Study the drawing (mm; zero at the part's minimum x, y, z) and answer. A direction names the side the tool comes from. Coordinates: 2 decimals unless noted, no trailing zeros. Loops run counter-clockwise (first coordinate to the right, second up) from the corner with the lowest first, then second, coordinate; pieces in that order, holes last. Notation, with made-up numbers: (63.25, 78.5) - (95.25, 78.5) arc R28 ccw to (95.25, 108.5) - close; hole circle Ø11 at (-1, 10). An arc over 180 degrees is marked (long way). Use one line per item in the form item = value.
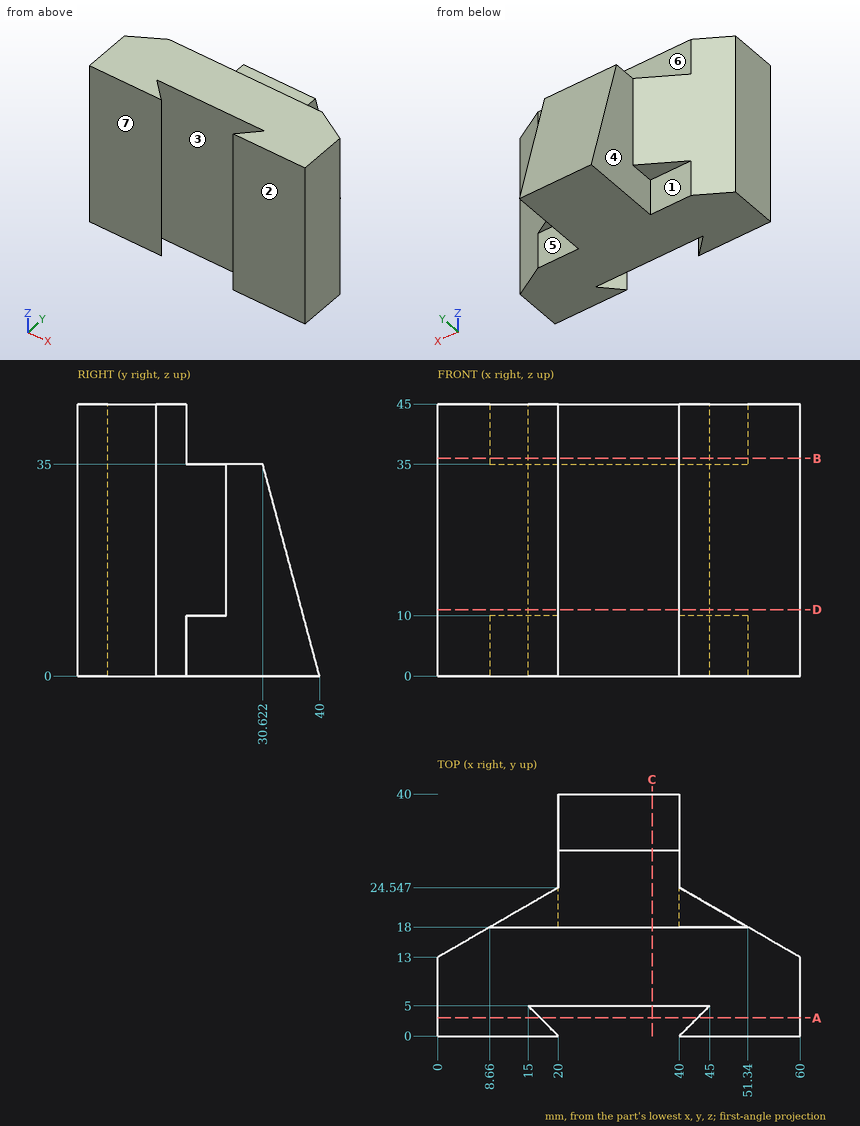
Item 1: The part is cut by section D-D on z = 11. Give the vertices of the cut face in (x, y).
Results below:
outline = (0, 0) - (20, 0) - (15, 5) - (45, 5) - (40, 0) - (60, 0) - (60, 13) - (40, 24.55) - (40, 37.05) - (20, 37.05) - (20, 24.55) - (0, 13) - close
Item 2: Each of these flat-tipped pins is pushed along its axis until it touches: P1, Ø2, axis at x = 46, y = 21.5, coming from the +Z side; P2, Ø1.5, axis at x = 11, z = 20, coming from the +Y side; P3, Ø17.5, axis at y = 28.5, z = 19.5, coming from the +X side. Where does it stop, or does it pass through?
Results below:
P1 = 35
P2 = 19.78
P3 = 48.31
Item 3: Which of the six approach directions +Z, -Z, +X, -X, +Y, -Y give full straight-line access (tool end or side, diameter ignored) to the marked faces 5, 6 and 7?
Results below:
face_5 = -Z, +X, +Y
face_6 = +Z, +X, -X, +Y
face_7 = +Z, -Z, +X, -X, -Y
Item 4: The part is cut by section C-C on x = 35.5. Give the vertices of the cut face in (y, z).
Results below:
outline = (5, 0) - (40, 0) - (30.62, 35) - (18, 35) - (18, 45) - (5, 45) - close
Item 5: The part is cut by section B-B on z = 36. Give the vertices of the cut face in (x, y).
Results below:
outline = (0, 0) - (20, 0) - (15, 5) - (45, 5) - (40, 0) - (60, 0) - (60, 13) - (51.34, 18) - (8.66, 18) - (0, 13) - close
Item 6: For a pull along Y with two mould halves and no side action, classify the marked faces 1, 2, 3 and 4 as +Y half, -Y half, draft (parallel to the pull), parting line (faces both ways), or undercut.
Results below:
face_1 = +Y half
face_2 = -Y half
face_3 = undercut
face_4 = draft
Item 7: Find the intervals of material crossed by L1, parallel to Y at x = 38.5, z = 40; L2, parallel to X at y = 2.5, z = 23; L3, parallel to Y at x = 44, z = 3, in increasing order.
Results below:
L1 = 5 to 18
L2 = 0 to 17.5, 42.5 to 60
L3 = 0 to 4, 5 to 18
Item 8: The part is cut by section A-A on y = 3. Give the vertices of the cut face in (x, z).
Results below:
outline = (0, 0) - (17, 0) - (17, 45) - (0, 45) - close; (43, 0) - (60, 0) - (60, 45) - (43, 45) - close
